from build123d import *

# Parameters (mm, degrees)
BOX_W             = 128
BOX_H             = 67
BOX_DEPTH         = 24
BOX001_W          = 116
BOX001_H          = 63
BOX001_DEPTH      = 22
BOX002_W          = 4
BOX002_H          = 34
BOX002_DEPTH      = 10
BOX003_W          = 100
BOX003_H          = 30
BOX003_DEPTH      = 1
BOX004_W          = 12
BOX004_H          = 32
BOX004_DEPTH      = 4
CYLINDER_R        = 3
CYLINDER_DEPTH    = 8
CYLINDER001_R     = 3
CYLINDER001_DEPTH = 8
CYLINDER002_R     = 1.5
CYLINDER002_DEPTH = 5
CYLINDER003_R     = 1.5
CYLINDER003_DEPTH = 5
BOX005_W          = 42
BOX005_H          = 20
BOX005_DEPTH      = 4
CYLINDER004_R     = 4
CYLINDER004_DEPTH = 6
CYLINDER005_R     = 4
CYLINDER005_DEPTH = 6
CYLINDER006_R     = 10
CYLINDER006_DEPTH = 4
CYLINDER007_R     = 8
CYLINDER007_DEPTH = 4
BOX006_W          = 10
BOX006_H          = 25
BOX006_DEPTH      = 1.5
BOX007_W          = 4
BOX007_H          = 7
BOX007_DEPTH      = 6
CYLINDER008_R     = 1.5
CYLINDER008_DEPTH = 2.5
CYLINDER009_R     = 1.5
CYLINDER009_DEPTH = 2.5
CYLINDER010_R     = 1
CYLINDER010_DEPTH = 5
CYLINDER011_R     = 1
CYLINDER011_DEPTH = 5
BOX008_W          = 18
BOX008_H          = 3
BOX008_DEPTH      = 6
BOX009_W          = 10
BOX009_H          = 5
BOX009_DEPTH      = 6
CYLINDER012_R     = 1.5
CYLINDER012_DEPTH = 5
CYLINDER013_R     = 1.5
CYLINDER013_DEPTH = 5
CYLINDER014_R     = 1.5
CYLINDER014_DEPTH = 5
CYLINDER015_R     = 1.5
CYLINDER015_DEPTH = 5
FILLET_R          = 1.5
CYLINDER016_R     = 5
CYLINDER016_DEPTH = 0.2
CYLINDER017_R     = 7
CYLINDER017_DEPTH = 0.2
CYLINDER018_R     = 7
CYLINDER018_DEPTH = 0.2
BOX010_W          = 5
BOX010_H          = 6
BOX010_DEPTH      = 0.2
BOX011_W          = 9
BOX011_H          = 4
BOX011_DEPTH      = 0.2
CYLINDER019_R     = 7
CYLINDER019_DEPTH = 0.2
CYLINDER020_R     = 5
CYLINDER020_DEPTH = 0.2
PRISM_DEPTH       = 0.2
CYLINDER021_R     = 1.8
CYLINDER021_DEPTH = 0.2


with BuildPart() as part:
    # Box → Box (join)
    with BuildSketch(Plane.XY):
        with Locations((64, 33.5)):
            Rectangle(BOX_W, BOX_H)
    extrude(amount=BOX_DEPTH)

    # Box001 → Box001 (cut)
    with BuildSketch(Plane(origin=(6, 2, 2), x_dir=(1, 0, 0), z_dir=(0, 0, 1))):
        with Locations((58, 31.5)):
            Rectangle(BOX001_W, BOX001_H)
    extrude(amount=BOX001_DEPTH, mode=Mode.SUBTRACT)

    # Box002 → Box002 (cut)
    with BuildSketch(Plane(origin=(122, 31, 2), x_dir=(1, 0, 0), z_dir=(0, 0, 1))):
        with Locations((2, 17)):
            Rectangle(BOX002_W, BOX002_H)
    extrude(amount=BOX002_DEPTH, mode=Mode.SUBTRACT)

    # Box003 → Box003 (cut)
    with BuildSketch(Plane(origin=(25, 34, 1), x_dir=(1, 0, 0), z_dir=(0, 0, 1))):
        with Locations((50, 15)):
            Rectangle(BOX003_W, BOX003_H)
    extrude(amount=BOX003_DEPTH, mode=Mode.SUBTRACT)

    # Box004 → Box004 (join)
    with BuildSketch(Plane(origin=(29, 2, 2), x_dir=(1, 0, 0), z_dir=(0, 0, 1))):
        with Locations((6, 16)):
            Rectangle(BOX004_W, BOX004_H)
    extrude(amount=BOX004_DEPTH)

    # Cylinder → Cylinder (join)
    with BuildSketch(Plane(origin=(35, 16, 6), x_dir=(1, 0, 0), z_dir=(0, 0, 1))):
        Circle(CYLINDER_R)
    extrude(amount=CYLINDER_DEPTH)

    # Cylinder001 → Cylinder001 (join)
    with BuildSketch(Plane(origin=(35, 31, 6), x_dir=(1, 0, 0), z_dir=(0, 0, 1))):
        Circle(CYLINDER001_R)
    extrude(amount=CYLINDER001_DEPTH)

    # Cylinder002 → Cylinder002 (cut)
    with BuildSketch(Plane(origin=(35, 31, 9), x_dir=(1, 0, 0), z_dir=(0, 0, 1))):
        Circle(CYLINDER002_R)
    extrude(amount=CYLINDER002_DEPTH, mode=Mode.SUBTRACT)

    # Cylinder003 → Cylinder003 (cut)
    with BuildSketch(Plane(origin=(35, 16, 9), x_dir=(1, 0, 0), z_dir=(0, 0, 1))):
        Circle(CYLINDER003_R)
    extrude(amount=CYLINDER003_DEPTH, mode=Mode.SUBTRACT)

    # Box005 → Box005 (cut)
    with BuildSketch(Plane(origin=(4, 50, 0), x_dir=(0, -1, 0), z_dir=(-1, 0, 0))):
        with Locations((21, 10)):
            Rectangle(BOX005_W, BOX005_H)
    extrude(amount=BOX005_DEPTH, mode=Mode.SUBTRACT)

    # Cylinder004 → Cylinder004 (cut)
    with BuildSketch(Plane(origin=(6, 50, 10), x_dir=(0, -1, 0), z_dir=(-1, 0, 0))):
        Circle(CYLINDER004_R)
    extrude(amount=CYLINDER004_DEPTH, mode=Mode.SUBTRACT)

    # Cylinder005 → Cylinder005 (cut)
    with BuildSketch(Plane(origin=(6, 9, 10), x_dir=(0, -1, 0), z_dir=(-1, 0, 0))):
        Circle(CYLINDER005_R)
    extrude(amount=CYLINDER005_DEPTH, mode=Mode.SUBTRACT)

    # Cylinder006 → Cylinder006 (cut)
    with BuildSketch(Plane(origin=(4, 50, 10), x_dir=(0, -1, 0), z_dir=(-1, 0, 0))):
        Circle(CYLINDER006_R)
    extrude(amount=CYLINDER006_DEPTH, mode=Mode.SUBTRACT)

    # Cylinder007 → Cylinder007 (cut)
    with BuildSketch(Plane(origin=(4, 9, 10), x_dir=(0, -1, 0), z_dir=(-1, 0, 0))):
        Circle(CYLINDER007_R)
    extrude(amount=CYLINDER007_DEPTH, mode=Mode.SUBTRACT)

    # Box006 → Box006 (join)
    with BuildSketch(Plane(origin=(74, 65, 6), x_dir=(0, 0, 1), z_dir=(0, -1, 0))):
        with Locations((5, 12.5)):
            Rectangle(BOX006_W, BOX006_H)
    extrude(amount=BOX006_DEPTH)

    # Box007 → Box007 (cut)
    with BuildSketch(Plane(origin=(65, 67.5, 9), x_dir=(0, 0, 1), z_dir=(0, -1, 0))):
        with Locations((2, 3.5)):
            Rectangle(BOX007_W, BOX007_H)
    extrude(amount=BOX007_DEPTH, mode=Mode.SUBTRACT)

    # Cylinder008 → Cylinder008 (cut)
    with BuildSketch(Plane(origin=(69, 66, 11), x_dir=(0, 0, 1), z_dir=(0, -1, 0))):
        Circle(CYLINDER008_R)
    extrude(amount=CYLINDER008_DEPTH, mode=Mode.SUBTRACT)

    # Cylinder009 → Cylinder009 (cut)
    with BuildSketch(Plane(origin=(55, 66, 11), x_dir=(0, 0, 1), z_dir=(0, -1, 0))):
        Circle(CYLINDER009_R)
    extrude(amount=CYLINDER009_DEPTH, mode=Mode.SUBTRACT)

    # Cylinder010 → Cylinder010 (join)
    with BuildSketch(Plane(origin=(123, 36, 1), x_dir=(-1, 0, 0), z_dir=(0, 0, 1))):
        Circle(CYLINDER010_R)
    extrude(amount=CYLINDER010_DEPTH)

    # Cylinder011 → Cylinder011 (join)
    with BuildSketch(Plane(origin=(123, 62, 1), x_dir=(-1, 0, 0), z_dir=(0, 0, 1))):
        Circle(CYLINDER011_R)
    extrude(amount=CYLINDER011_DEPTH)

    # Box008 → Box008 (cut)
    with BuildSketch(Plane(origin=(122, 24.5, 21), x_dir=(0, 1, 0), z_dir=(1, 0, 0))):
        with Locations((9, 1.5)):
            Rectangle(BOX008_W, BOX008_H)
    extrude(amount=BOX008_DEPTH, mode=Mode.SUBTRACT)

    # Box009 → Box009 (cut)
    with BuildSketch(Plane(origin=(122, 28.5, 16), x_dir=(0, 1, 0), z_dir=(1, 0, 0))):
        with Locations((5, 2.5)):
            Rectangle(BOX009_W, BOX009_H)
    extrude(amount=BOX009_DEPTH, mode=Mode.SUBTRACT)

    # Cylinder012 → Cylinder012 (cut)
    with BuildSketch(Plane(origin=(3, 3, 19), x_dir=(0, -1, 0), z_dir=(0, 0, 1))):
        Circle(CYLINDER012_R)
    extrude(amount=CYLINDER012_DEPTH, mode=Mode.SUBTRACT)

    # Cylinder013 → Cylinder013 (cut)
    with BuildSketch(Plane(origin=(3, 64, 19), x_dir=(0, -1, 0), z_dir=(0, 0, 1))):
        Circle(CYLINDER013_R)
    extrude(amount=CYLINDER013_DEPTH, mode=Mode.SUBTRACT)

    # Cylinder014 → Cylinder014 (cut)
    with BuildSketch(Plane(origin=(125, 64, 19), x_dir=(0, -1, 0), z_dir=(0, 0, 1))):
        Circle(CYLINDER014_R)
    extrude(amount=CYLINDER014_DEPTH, mode=Mode.SUBTRACT)

    # Cylinder015 → Cylinder015 (cut)
    with BuildSketch(Plane(origin=(125, 3, 19), x_dir=(0, -1, 0), z_dir=(0, 0, 1))):
        Circle(CYLINDER015_R)
    extrude(amount=CYLINDER015_DEPTH, mode=Mode.SUBTRACT)

    # Fillet
    fillet_edges = [part.edges().sort_by_distance(p)[0] for p in [
        (128, 0, 12),
        (128, 33.5, 0),
        (128, 67, 12),
        (64, 67, 0),
        (64, 0, 0),
        (0, 67, 12),
        (0, 0, 12),
    ]]
    fillet(fillet_edges, radius=FILLET_R)

    # Cylinder016 → Cylinder016 (cut)
    with BuildSketch(Plane(origin=(68, 24, 1.8), x_dir=(0, -1, 0), z_dir=(0, 0, 1))):
        Circle(CYLINDER016_R)
    extrude(amount=CYLINDER016_DEPTH, mode=Mode.SUBTRACT)

    # Cylinder017 → Cylinder017 (cut)
    with BuildSketch(Plane(origin=(70, 14, 1.8), x_dir=(0, -1, 0), z_dir=(0, 0, 1))):
        Circle(CYLINDER017_R)
    extrude(amount=CYLINDER017_DEPTH, mode=Mode.SUBTRACT)

    # Cylinder018 → Cylinder018 (cut)
    with BuildSketch(Plane(origin=(74, 14, 1.8), x_dir=(0, -1, 0), z_dir=(0, 0, 1))):
        Circle(CYLINDER018_R)
    extrude(amount=CYLINDER018_DEPTH, mode=Mode.SUBTRACT)

    # Box010 → Box010 (cut)
    with BuildSketch(Plane(origin=(69, 12, 1.8), x_dir=(0, -1, 0), z_dir=(0, 0, 1))):
        with Locations((2.5, 3)):
            Rectangle(BOX010_W, BOX010_H)
    extrude(amount=BOX010_DEPTH, mode=Mode.SUBTRACT)

    # Box011 → Box011 (cut)
    with BuildSketch(Plane(origin=(76.1, 22, 1.8), x_dir=(0.104528, -0.994522, 0), z_dir=(0, 0, 1))):
        with Locations((4.5, 2)):
            Rectangle(BOX011_W, BOX011_H)
    extrude(amount=BOX011_DEPTH, mode=Mode.SUBTRACT)

    # Cylinder019 → Cylinder019 (join)
    with BuildSketch(Plane(origin=(74.791893, 24.879037, 1.8), x_dir=(0.104528, -0.994522, 0), z_dir=(0, 0, 1))):
        Circle(CYLINDER019_R)
    extrude(amount=CYLINDER019_DEPTH)

    # Cylinder020 → Cylinder020 (cut)
    with BuildSketch(Plane(origin=(67.830239, 24.147338, 1.8), x_dir=(0.104528, -0.994522, 0), z_dir=(0, 0, 1))):
        Circle(CYLINDER020_R)
    extrude(amount=CYLINDER020_DEPTH, mode=Mode.SUBTRACT)

    # Prism → Prism (cut)
    with BuildSketch(Plane(origin=(62.360369, 23.572431, 1.8), x_dir=(0.5, -0.866025, 0), z_dir=(0, 0, 1))):
        Polygon((2.5, 0), (-1.25, 2.165064), (-1.25, -2.165064), align=None)
    extrude(amount=PRISM_DEPTH, mode=Mode.SUBTRACT)

    # Cylinder021 → Cylinder021 (join)
    with BuildSketch(Plane(origin=(61.187164, 25.204482, 1.8), x_dir=(0.5, -0.866025, 0), z_dir=(0, 0, 1))):
        Circle(CYLINDER021_R)
    extrude(amount=CYLINDER021_DEPTH)


solid = part.part
Could you check a few things on this model? Use its own coordinates, in mm. A direction names the side the tool comes from. Give positions to 0.01 mm unless a question says otherwise; leave off trailing zeros. Order: outer loops, then holes, each group sorted by start corner. A loop starts at its lowest first (then second) coordinate and runs counter-clockwise, first axis right, second up.
Item 1: If we section it at A-A, the plane z = 4.25: Write out the boundary of the cut face in (x, y), plus the area to 3 significant figures.
Item 2: If we mould it in two halves opening along Z, with no side actions, what happens to faces 4 (the face through (3, 3, 19)), 5 (the face through (128, 33, 13)), 6 (the face through (62, 65, 9))? For each: pulls with the +Z half, pulls with the -Z half, needs draft (parallel to the pull), parting line crosses it, or undercut.
Item 3: If we section it at D-D, the plane y = 58.5: Write out the boundary of the cut face in (x, z), plus the area to 3 significant figures.
Item 4: I need wall thicknesses on line 1 (Y direction, x = 125, z = 20.15); line 2 (X direction, y = 3, z = 22.7); line 3 (Y direction, x = 35, z = 10.85). Which ranges of each line are inside material? Lowest first, please.
Item 5: For faces 1 (the face through (5, 54, 10)), 2 (the face through (126.487, 3.195, 21.465)), 3 (the face through (125, 40, 21)), which set-ups out of +Z, -Z, +X, -X, +Y, -Y let a thin tool reach every point of the face, with its end or its side?
Item 6: If we section it at B-B, the plane x = 30.5: Write out the boundary of the cut face in (y, z), plus the area to 3 significant figures.
Item 7: If we section it at C-C, the plane z = 22.25: Write out the boundary of the cut face in (x, y), plus the area to 3 significant figures.
Item 8: I'm going to push flat-ended pins straight in: pin 1 (1.2 mm diameter, centred on x = 125.5, y = 41, fed in from +Z); pin 2 (6.5 mm diameter, centred on x = 34.5, y = 17, fed in from +Z); pin 3 (7 mm diameter, centred on y = 9, z = 10, fed in from -X). Where does each tip first touch, or does it pass through?
Values:
1. outline: (0, 1.5) arc R1.5 ccw to (1.5, 0) - (126.5, 0) arc R1.5 ccw to (128, 1.5) - (128, 65.5) arc R1.5 ccw to (126.5, 67) - (1.5, 67) arc R1.5 ccw to (0, 65.5) - (0, 58.18) - (4, 58.18) - (4, 3.44) - (0, 3.44) - close; circle Ø2 at (123, 36); circle Ø2 at (123, 62); hole (6, 2) - (29, 2) - (29, 34) - (41, 34) - (41, 2) - (122, 2) - (122, 31) - (126, 31) - (126, 65) - (6, 65) - close
1. area: 1,300 mm2
2. face 4: pulls with the +Z half
2. face 5: needs draft
2. face 6: undercut
3. outline: (0, 0) - (126.5, 0) arc R1.5 ccw to (128, 1.5) - (128, 24) - (122, 24) - (122, 12) - (126, 12) - (126, 2) - (125, 2) - (125, 1) - (25, 1) - (25, 2) - (6, 2) - (6, 24) - (0, 24) - (0, 15.27) - (4, 15.27) - (4, 4.73) - (0, 4.73) - close
3. area: 337 mm2
4. line 1: y = 0 to 1.5, 4.5 to 28.5, 38.5 to 62.5, 65.5 to 67
4. line 2: x = 0 to 1.5, 4.5 to 6, 122 to 123.5, 126.5 to 128
4. line 3: y = 0 to 2, 13 to 14.5, 17.5 to 19, 28 to 29.5, 32.5 to 34, 65 to 67
5. face 1: -X
5. face 2: +Z
5. face 3: +Z, +X
6. outline: (0, 1.5) arc R1.5 ccw to (1.5, 0) - (65.5, 0) arc R1.5 ccw to (67, 1.5) - (67, 24) - (65, 24) - (65, 2) - (64, 2) - (64, 1) - (34, 1) - (34, 6) - (2, 6) - (2, 24) - (0, 24) - close
6. area: 319 mm2
7. outline: (0, 1.5) arc R1.5 ccw to (1.5, 0) - (126.5, 0) arc R1.5 ccw to (128, 1.5) - (128, 24.5) - (122, 24.5) - (122, 2) - (6, 2) - (6, 65) - (122, 65) - (122, 42.5) - (128, 42.5) - (128, 65.5) arc R1.5 ccw to (126.5, 67) - (1.5, 67) arc R1.5 ccw to (0, 65.5) - close; hole circle Ø3 at (3, 3); hole circle Ø3 at (3, 64); hole circle Ø3 at (125, 3); hole circle Ø3 at (125, 64)
7. area: 1,130 mm2
8. pin 1: stops at z = 21
8. pin 2: stops at z = 14
8. pin 3: stops at x = 122
